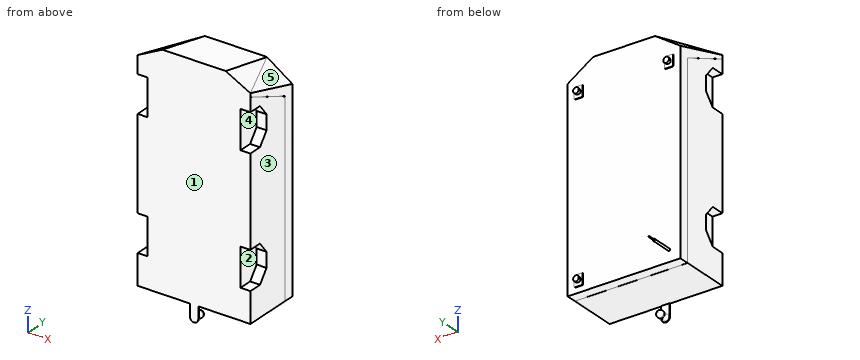
from build123d import *

# Parameters (mm, degrees)
CROQUIS1_W              = 800
CROQUIS1_H              = 1600
SALIENTE_EXTRUIR1_DEPTH = 415
CORTAR_EXTRUIR1_DEPTH   = 200
CORTAR_EXTRUIR2_DEPTH   = 200
CORTAR_EXTRUIR6_DEPTH   = 499
CORTAR_EXTRUIR8_DEPTH   = 359
CORTAR_EXTRUIR10_DEPTH  = 353
CORTAR_EXTRUIR12_DEPTH  = 514
CORTAR_EXTRUIR13_DEPTH  = 514
CORTAR_EXTRUIR16_DEPTH  = 70
CORTAR_EXTRUIR17_DEPTH  = 70
CORTAR_EXTRUIR18_DEPTH  = 1
CROQUIS20_W             = 800
CROQUIS20_H             = 1
CORTAR_EXTRUIR19_DEPTH  = 1
SALIENTE_EXTRUIR2_DEPTH = 5
CROQUIS22_R             = 15
SALIENTE_EXTRUIR3_DEPTH = 10
CROQUIS23_R             = 20
SALIENTE_EXTRUIR4_DEPTH = 15
SALIENTE_EXTRUIR5_DEPTH = 5
CROQUIS26_R             = 25
SALIENTE_EXTRUIR6_DEPTH = 75
CROQUIS30_W             = 3.75
CROQUIS30_H             = 50


with BuildPart() as part:
    # Croquis1 → Saliente-Extruir1 (new body)
    with BuildSketch(Plane(origin=(0, 0, 0), x_dir=(1, 0, 0), z_dir=(0, 1, 0))):
        with Locations((0, -407.98258177)):
            Rectangle(CROQUIS1_W, CROQUIS1_H)
    extrude(amount=SALIENTE_EXTRUIR1_DEPTH)

    # Croquis3 → Cortar-Extruir1 (cut)
    with BuildSketch(Plane(origin=(604.100569287, 262.019524028, 906.150853931), x_dir=(-0.8421068082275548, 0.1498081502111445, 0.5180865194802076), z_dir=(-0.5393107856670403, -0.23391793113269235, -0.8089661785005605))):
        Polygon((456.118589156, 88.118028239), (242.368981337, -310.549885139), (242.368981337, 121.451272267), align=None)
    extrude(amount=-CORTAR_EXTRUIR1_DEPTH, mode=Mode.SUBTRACT)

    # Croquis5 → Cortar-Extruir2 (cut)
    with BuildSketch(Plane(origin=(-604.100569287, 262.019524028, 906.150853931), x_dir=(-0.8421068082275548, -0.1498081502111445, -0.5180865194802076), z_dir=(0.5393107856670404, -0.2339179311326923, -0.8089661785005605))):
        Polygon((-242.368981337, -310.549885139), (-242.368981337, 121.451272267), (-456.118589156, 88.118028239), align=None)
    extrude(amount=-CORTAR_EXTRUIR2_DEPTH, mode=Mode.SUBTRACT)

    # Croquis8 → Cortar-Extruir6 (cut)
    with BuildSketch(Plane(origin=(0, 250.204627362, 1153.721337281), x_dir=(-1, 0, 0), z_dir=(0, -0.21194078521367435, -0.9772825095963864))):
        Polygon((220, 168.626135247), (400, -256.020776905), (-400, -256.020776905), (-220, 168.626135247), (0, 168.626135247), align=None)
    extrude(amount=-CORTAR_EXTRUIR6_DEPTH, mode=Mode.SUBTRACT)

    # Croquis12 → Cortar-Extruir8 (cut)
    with BuildSketch(Plane.XY.offset(1117.98258177)):
        Polygon((220, 415), (400, 0), (400, 415), align=None)
    extrude(amount=CORTAR_EXTRUIR8_DEPTH, mode=Mode.SUBTRACT)

    # Croquis14 → Cortar-Extruir10 (cut)
    with BuildSketch(Plane.XY.offset(1117.98258177)):
        Polygon((-220, 415), (-400, 0), (-400, 415), align=None)
    extrude(amount=CORTAR_EXTRUIR10_DEPTH, mode=Mode.SUBTRACT)

    # Croquis15 → Cortar-Extruir12 (cut)
    with BuildSketch(Plane(origin=(516.98244579, 224.233349981, 1008.11576929), x_dir=(-0.8942171635698928, 0.0971910742249457, 0.4369548712029846), z_dir=(-0.44763340400043405, -0.19415424751826063, -0.8728851378008463))):
        Polygon((327.082120211, -262.279632659), (130.821069596, -242.738649788), (332.114454842, 162.361304614), align=None)
    extrude(amount=-CORTAR_EXTRUIR12_DEPTH, mode=Mode.SUBTRACT)


with BuildPart() as body_2:
    # of the pieces the cut leaves, the one that is kept (cortar_extruir12_keep)
    add(part.part.solids().sort_by_distance((-400, 0, 1207.98258177))[0])

    # Croquis16 → Cortar-Extruir13 (cut)
    with BuildSketch(Plane(origin=(-516.98244579, 224.233349981, 1008.11576929), x_dir=(-0.8942171635698928, -0.09719107422494568, -0.43695487120298454), z_dir=(0.44763340400043394, -0.19415424751826066, -0.8728851378008463))):
        Polygon((-327.082120211, -262.279632659), (-332.114454842, 162.361304614), (-130.821069596, -242.738649788), align=None)
    extrude(amount=-CORTAR_EXTRUIR13_DEPTH, mode=Mode.SUBTRACT)


with BuildPart() as body_2_2:
    # of the pieces the cut leaves, the one that is kept (cortar_extruir13_keep)
    add(body_2.part.solids().sort_by_distance((224.5, 0, 1207.98258177))[0])

    # Croquis17 → Cortar-Extruir16 (cut)
    with BuildSketch(Plane(origin=(400, 0, 0), x_dir=(0, 0, -1), z_dir=(1, 0, 0))):
        Polygon((177.01741823, 0), (-92.98258177, 0), (-92.98258177, 95), (-10.48258177, 160), (94.51741823, 160), (177.01741823, 95), align=None)
        Polygon((-992.98258177, 0), (-722.98258177, 0), (-722.98258177, 95), (-805.48258177, 160), (-910.48258177, 160), (-992.98258177, 95), align=None)
    extrude(amount=-CORTAR_EXTRUIR16_DEPTH, mode=Mode.SUBTRACT)

    # Croquis18 → Cortar-Extruir17 (cut)
    with BuildSketch(Plane.ZY.offset(400)):
        Polygon((-177.01741823, 0), (82.98258177, 0), (82.98258177, 95), (5.48258177, 160), (-99.51741823, 160), (-177.01741823, 95), align=None)
        Polygon((992.98258177, 0), (732.98258177, 0), (732.98258177, 95), (810.48258177, 160), (915.48258177, 160), (992.98258177, 95), align=None)
    extrude(amount=-CORTAR_EXTRUIR17_DEPTH, mode=Mode.SUBTRACT)

    # Croquis19 → Cortar-Extruir18 (cut)
    with BuildSketch(Plane(origin=(400, 0, 0), x_dir=(0, 0, -1), z_dir=(1, 0, 0))):
        Polygon((392.01741823, 343), (-948.718987098, 343), (-1091.223533976, 0), (-1092.306405756, 0), (-949.386393727, 344), (392.01741823, 344), align=None)
    cortar_extruir18 = extrude(amount=-CORTAR_EXTRUIR18_DEPTH, mode=Mode.SUBTRACT)

    # Croquis20 → Cortar-Extruir19 (cut)
    with BuildSketch(Plane(origin=(0, 0, -392.01741823), x_dir=(-1, 0, 0), z_dir=(0, 0, -1))):
        with Locations((0, 343.5)):
            Rectangle(CROQUIS20_W, CROQUIS20_H)
    extrude(amount=-CORTAR_EXTRUIR19_DEPTH, mode=Mode.SUBTRACT)

    # Simetr_a1: Cortar-Extruir18 across plane
    add(cortar_extruir18.mirror(Plane.ZY), mode=Mode.SUBTRACT)

    # Croquis21 → Saliente-Extruir2 (add)
    with BuildSketch(Plane(origin=(0, 415, 0), x_dir=(1, 0, 0), z_dir=(0, 1, 0))):
        with BuildLine():
            Line((295, 272.01741823), (345, 272.01741823))
            ThreePointArc((345, 272.01741823), (348.535533906, 273.481884325), (350, 277.01741823))
            Line((350, 277.01741823), (350, 347.01741823))
            ThreePointArc((350, 347.01741823), (348.535533906, 350.552952136), (345, 352.01741823))
            Line((345, 352.01741823), (295, 352.01741823))
            ThreePointArc((295, 352.01741823), (291.464466094, 350.552952136), (290, 347.01741823))
            Line((290, 347.01741823), (290, 277.01741823))
            ThreePointArc((290, 277.01741823), (291.464466094, 273.481884325), (295, 272.01741823))
        make_face()
        with BuildLine():
            Line((290, -882.98258177), (290, -952.98258177))
            ThreePointArc((290, -952.98258177), (291.464466094, -956.518115675), (295, -957.98258177))
            Line((295, -957.98258177), (345, -957.98258177))
            ThreePointArc((345, -957.98258177), (348.535533906, -956.518115675), (350, -952.98258177))
            Line((350, -952.98258177), (350, -882.98258177))
            ThreePointArc((350, -882.98258177), (348.535533906, -879.447047864), (345, -877.98258177))
            Line((345, -877.98258177), (295, -877.98258177))
            ThreePointArc((295, -877.98258177), (291.464466094, -879.447047864), (290, -882.98258177))
        make_face()
        with BuildLine():
            Line((-295, -877.98258177), (-345, -877.98258177))
            ThreePointArc((-345, -877.98258177), (-348.535533906, -879.447047864), (-350, -882.98258177))
            Line((-350, -882.98258177), (-350, -952.98258177))
            ThreePointArc((-350, -952.98258177), (-348.535533906, -956.518115675), (-345, -957.98258177))
            Line((-345, -957.98258177), (-295, -957.98258177))
            ThreePointArc((-295, -957.98258177), (-291.464466094, -956.518115675), (-290, -952.98258177))
            Line((-290, -952.98258177), (-290, -882.98258177))
            ThreePointArc((-290, -882.98258177), (-291.464466094, -879.447047864), (-295, -877.98258177))
        make_face()
    extrude(amount=SALIENTE_EXTRUIR2_DEPTH)

    # Croquis22 → Saliente-Extruir3 (add)
    with BuildSketch(Plane(origin=(0, 420, 0), x_dir=(1, 0, 0), z_dir=(0, 1, 0))):
        with Locations(Location((320, 312.01741823, 0), (0, 0, 270))):
            Circle(CROQUIS22_R)
        with Locations(Location((320, -917.98258177, 0), (0, 0, 270))):
            Circle(CROQUIS22_R)
        with Locations(Location((-320, -917.98258177, 0), (0, 0, 90))):
            Circle(CROQUIS22_R)
    extrude(amount=SALIENTE_EXTRUIR3_DEPTH)

    # Croquis23 → Saliente-Extruir4 (add)
    with BuildSketch(Plane(origin=(0, 430, 0), x_dir=(1, 0, 0), z_dir=(0, 1, 0))):
        with Locations(Location((320, 312.01741823, 0), (0, 0, 270))):
            Circle(CROQUIS23_R)
        with Locations(Location((320, -917.98258177, 0), (0, 0, 270))):
            Circle(CROQUIS23_R)
        with Locations(Location((-320, -917.98258177, 0), (0, 0, 270))):
            Circle(CROQUIS23_R)
    extrude(amount=SALIENTE_EXTRUIR4_DEPTH)

    # Croquis25 → Saliente-Extruir5 (add)
    with BuildSketch(Plane.XZ):
        with BuildLine():
            Line((-30, -476.764876907), (-30, -392.01741823))
            Line((-30, -392.01741823), (30, -392.01741823))
            Line((30, -392.01741823), (30, -476.764876907))
            ThreePointArc((30, -476.764876907), (0, -506.764876907), (-30, -476.764876907))
        make_face()
    extrude(amount=-SALIENTE_EXTRUIR5_DEPTH)

    # Croquis26 → Saliente-Extruir6 (add)
    with BuildSketch(Plane(origin=(0, 5, 0), x_dir=(1, 0, 0), z_dir=(0, 1, 0))):
        with Locations(Location((0, 476.764876907, 0), (0, 0, 90))):
            Circle(CROQUIS26_R)
    extrude(amount=SALIENTE_EXTRUIR6_DEPTH)

    # Croquis28 → Cortar-Revoluci_n7 (revolve, cut)
    with BuildSketch(Plane.ZY):
        with BuildLine():
            ThreePointArc((-451.764876907, 55), (-454.267783945, 44.096752398), (-461.275341569, 35.376690009))
            add(Edge.make_bspline(
                [(-461.275341569, 35.376690009), (-479.429840017, 14.56995995), (-453.764876907, 5)],
                knots=[0, 0, 0, 1, 1, 1], degree=2))
            Line((-453.764876907, 5), (-451.764876907, 5))
            Line((-451.764876907, 5), (-451.764876907, 55))
        make_face()
    revolve(axis=Axis((0, 90.386786237, -476.764876907), (0, -1, 0)), mode=Mode.SUBTRACT)

    # Croquis29 → Cortar-Revoluci_n26 (revolve, cut)
    with BuildSketch(Plane.ZY):
        with BuildLine():
            Line((-475.149447102, 80), (-475.149447102, 84.514502028))
            Line((-475.149447102, 84.514502028), (-446.334832781, 84.514502028))
            Line((-446.334832781, 84.514502028), (-446.334832781, 57.478552518))
            Line((-446.334832781, 57.478552518), (-451.764876907, 56.615429804))
            ThreePointArc((-451.764876907, 56.615429804), (-459.050340313, 72.714536594), (-475.149447102, 80))
        make_face()
    revolve(axis=Axis((0, 80, -476.764876907), (0, -1, 0)), mode=Mode.SUBTRACT)

    # Croquis30 → Revoluci_n1 (revolve)
    with BuildSketch(Plane(origin=(0, 0, -312.01741823), x_dir=(-1, 0, 0), z_dir=(0, 0, -1)), mode=Mode.PRIVATE) as revoluci_n1_sk:
        with Locations((321.875, 590)):
            Rectangle(CROQUIS30_W, CROQUIS30_H)
        Polygon((320, 415), (320, 565), (323.75, 565), (327.5, 565), (327.5, 415), align=None)
    revolve(revoluci_n1_sk.sketch.rotate(Axis((-320, 633.577098179, -312.01741823), (0, -1, 0)), 270), axis=Axis((-320, 633.577098179, -312.01741823), (0, -1, 0)))


solid = body_2_2.part
Can you work these out from the model? Positions are in its coordinate system, mm. Face numbers are marked on the shaded views. A direction names the side the tool comes from. Round coordinates to 2 decimals unless told otherwise and drop trailing zeros. Loops run counter-clockwise (first coordinate to the right, second up) from the corner with the lowest first, then second, coordinate; pieces in that order, holes last. Notation, with made-up numbers: (2, 58.5) - (54, 58.5) arc R25 cw to (54, 89.5) - close; hole circle Ø10 at (51.25, 60). An arc over 180 degrees is marked (long way). Use CSV: the item, a comma, the result in double quotes. Start each with the question number.
1) If we section it at A-A on x = -142: Write out the boundary of the cut face in (y, z), plus the area to 3 significant figures.
2) If we section it at C-C on y = 246: Write out the boundary of the cut face in (x, z), plus the area to 3 significant figures.
3) If we section it at D-D on x = 246.5: Write out the boundary of the cut face in (y, z).
4) For the marked faces 1 and 2, which set-ups out of +Z, -Z, +X, -X, +Y, -Y let a thin tool reach every point of the face, with its end or its side?
5) For pin 1 Ø4 at (x, z) = (-314, 952.5) entering from +Y; pin 2 Ø12 at (x, z) = (-323.5, 919) entering from +Y; pin 3 Ø1 at (x, z) = (-0.5, -477.5) entering from +Y, each with a flat end and sliding along its axis, tell me the tip position at first contact or that it passes through.
6) If we section it at B-B on z = 757: Write out the boundary of the cut face in (x, y), plus the area to 3 significant figures.
7) Please list where these lines run through material, in increasing order: probe 1 along Y at (x, z) = (-142.5, 655); probe 2 along Z at (x, y) = (157.5, 49.5); probe 3 along Z at (x, y) = (1, 189). Write a range as [from, to].
8) We'd pull the mould along Z, two halves only. Please class the marked faces 3, 4 and 5: released by +Z, released by -Z, zero draft, split by the parting line, or undercut.
Geometry results:
1,outline,"(0, -392.02) - (343, -392.02) - (343, -391.02) - (344, -391.02) - (344, -392.02) - (415, -392.02) - (415, 1117.98) - (0, 1207.98) - close"
1,area,"645,000 mm2"
2,outline,"(-400, -392.02) - (400, -392.02) - (400, 989.02) - (399, 989.02) - (399, 990.1) - (400, 990.1) - (400, 1046.85) - (293.3, 1117.98) - (221.83, 1154.63) - (-221.83, 1154.63) - (-293.3, 1117.98) - (-400, 1046.85) - (-400, 990.1) - (-399, 990.1) - (-399, 989.02) - (-400, 989.02) - close"
2,area,"1,220,000 mm2"
3,outline,"(0, -392.02) - (343, -392.02) - (343, -391.02) - (344, -391.02) - (344, -392.02) - (415, -392.02) - (415, 1100.32) - (353.9, 1117.98) - (0, 1196.7) - close"
4,face 1,"+Z, -Z, +X, -X, -Y"
4,face 2,"+X, -Y"
5,pin 1,"stops at y = 420"
5,pin 2,"stops at y = 445"
5,pin 3,"stops at y = 80"
6,outline,"(-400, 115.14) - (-330, 115.14) - (-330, 0) - (330, 0) - (330, 121.8) - (400, 121.8) - (400, 343) - (399, 343) - (399, 344) - (400, 344) - (400, 415) - (-400, 415) - (-400, 344) - (-399, 344) - (-399, 343) - (-400, 343) - close"
6,area,"315,000 mm2"
7,probe 1,"y = [0, 415]"
7,probe 2,"z = [-392.02, 1197.25]"
7,probe 3,"z = [-392.02, 1166.99]"
8,face 3,"zero draft"
8,face 4,"undercut"
8,face 5,"released by +Z"
